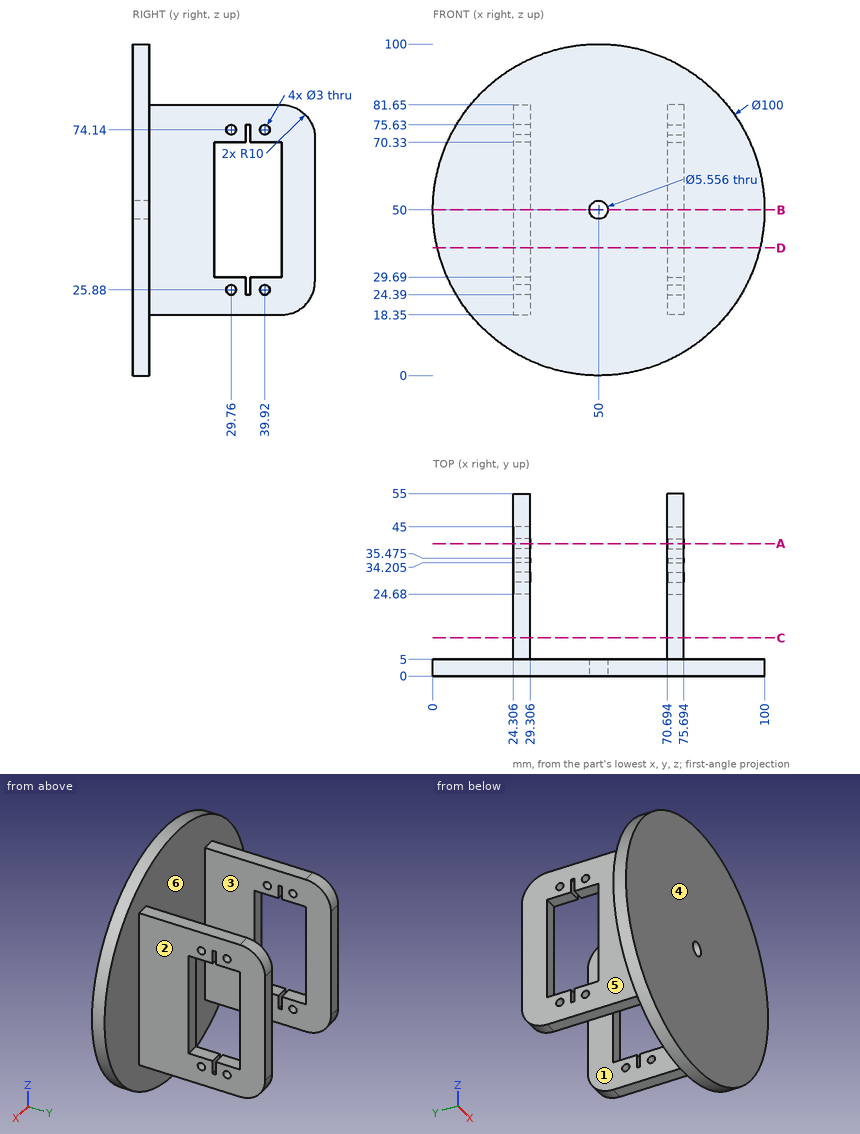
Job drawing, mm, ordinate dimensions from the low corner. One solid piece. A direction names the side the tool comes from. Give positions to 0.01 mm unless a question says otherwise; leave off trailing zeros. Loops run counter-clockwise (first coordinate to the right, second up) from the corner with the lowest first, then second, coordinate; pieces in that order, holes last. Notation, with made-up numbers: (38, 69.5) - (94, 69.5) arc R30 ccw to (94, 91.5) - close; hole circle Ø11 at (3.5, 36). An arc over 180 degrees is marked (long way). Use one line per item in the form item = value.
(1) Pull direction X, two halves, no side cores. Call the marked faces 3, 4, 5 and 6: pulls with the +X half, pulls with the -X half, needs draft (parallel to the pull), parting line crosses it, or undercut.
Determined:
face_3 = undercut
face_4 = needs draft
face_5 = pulls with the -X half
face_6 = undercut
(2) Drop flat-ended pins along their axis: P1, Ø1.5, axis at x = 73, y = 31, coming from the -Z side; P2, Ø1.4, axis at x = 73, y = 35, coming from the +Z side; P3, Ø5.5, axis at x = 74.5, z = 26.5, coming from the -Y side; P4, Ø6, axis at y = 35, z = 71, coming from the +X side. Give the stop position or say it passes through.
Determined:
P1 = 18.35
P2 = 81.65
P3 = 0
P4 = 75.69
(3) Cut at A-A (y = 39.92). Count the separate pieces of the cut face and the enclosed holes in it, then the cut area to 3 significant figures.
Determined:
separate_pieces = 8
enclosed_holes = 0
area = 167 mm^2
(4) Cut at B-B (z = 50). Give the cut face in (x, y), then the cut area to 3 significant figures.
Determined:
outline = (0, 0) - (47.22, 0) - (47.22, 5) - (29.31, 5) - (29.31, 24.68) - (24.31, 24.68) - (24.31, 5) - (0, 5) - close; (24.31, 45) - (29.31, 45) - (29.31, 55) - (24.31, 55) - close; (52.78, 0) - (100, 0) - (100, 5) - (75.69, 5) - (75.69, 24.68) - (70.69, 24.68) - (70.69, 5) - (52.78, 5) - close; (70.69, 45) - (75.69, 45) - (75.69, 55) - (70.69, 55) - close
area = 769 mm^2
(5) 3-axis set-ups, long thin cutter, end or side, ignore diameter. For the marked faces 1 and 2: which of +Z, -Z, +X, -X, +Y, -Y reach the whole face in a straight line?
Determined:
face_1 = +Z, -Z, +Y
face_2 = +Z, -Z, +X, +Y
(6) Cut at D-D (z = 38.5). Give the cut face in (x, y).
Determined:
outline = (1.34, 0) - (98.66, 0) - (98.66, 5) - (75.69, 5) - (75.69, 24.68) - (70.69, 24.68) - (70.69, 5) - (29.31, 5) - (29.31, 24.68) - (24.31, 24.68) - (24.31, 5) - (1.34, 5) - close; (24.31, 45) - (29.31, 45) - (29.31, 55) - (24.31, 55) - close; (70.69, 45) - (75.69, 45) - (75.69, 55) - (70.69, 55) - close
(7) Drill centre lines: L1, parallel to Z at x = 73.5, y = 29.76; L2, parallel to Y at x = 73.3, z = 74.14 (1 decimal); L3, parallel to Z at x = 26, y = 29. Where is each one in solid material? Low to high.
Determined:
L1 = 18.35 to 24.38, 27.38 to 29.69, 70.33 to 72.64, 75.64 to 81.65
L2 = 0 to 28.3, 31.3 to 34.2, 35.5 to 38.4, 41.4 to 54.7
L3 = 18.35 to 24.59, 27.17 to 29.69, 70.33 to 72.85, 75.43 to 81.65
(8) Cut at C-C (y = 11.5). Give the cut face in (x, z), then the cut area to 3 significant figures.
Determined:
outline = (24.31, 18.35) - (29.31, 18.35) - (29.31, 81.65) - (24.31, 81.65) - close; (70.69, 18.35) - (75.69, 18.35) - (75.69, 81.65) - (70.69, 81.65) - close
area = 633 mm^2
